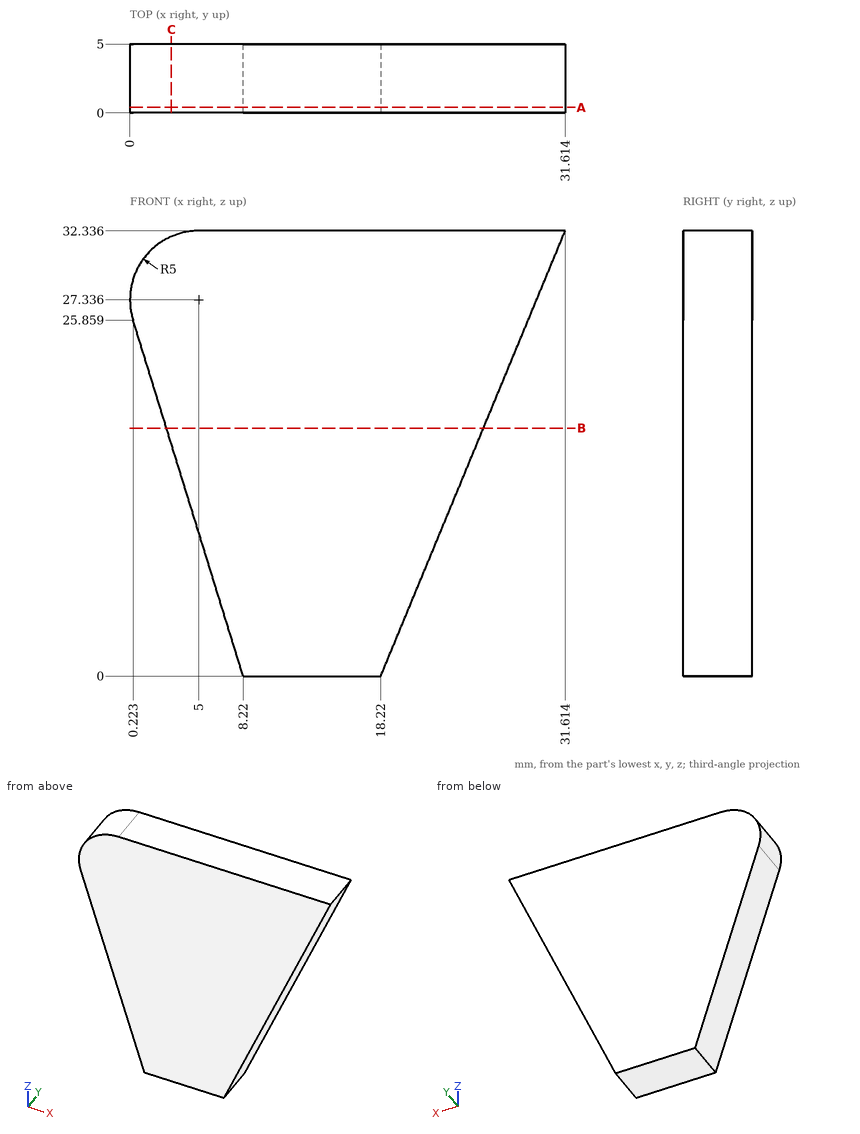
Study the drawing (mm; zero at the part's minimum x, y, z) and answer. Give positions to 0.01 mm unless a question says otherwise; leave off trailing zeros. Write each loop counter-clockwise with the first axis right and the second up, starting at its lowest first coordinate (ties: lowest second). Pieces come first, ordered by that corner, then holes.
(1) Flat-ended cylindrical pins translate along their axes: pin 1 Ø1.5 at (y, z) = (2, 25) entering from -X; pin 2 Ø2 at (y, z) = (4.5, 7.5) entering from +X; pin 3 Ø1 at (y, z) = (3, 8) entering from -X. Find the tip coordinate at first contact, or state that the pin passes through.
Final values:
pin 1: stops at x = 0.26
pin 2: stops at x = 21.74
pin 3: stops at x = 5.59
(2) Straight lines are drawn through the part: line 1 (X direction, y = 1.4, z = 18) (1 decimal); line 2 (Z direction, x = 24.5, y = 2.85) (1 decimal); line 3 (Z direction, x = 22, y = 0.75) (1 decimal). For each, find the intervals that lie inside material, in ascending order.
Final values:
line 1: x = 2.7 to 25.7
line 2: z = 15.2 to 32.3
line 3: z = 9.1 to 32.3
(3) The part is cut by section A-A on y = 0.4. Write down the section's boundary in (x, z) (1 decimal), plus the area to 3 significant figures.
Final values:
outline: (0.2, 25.9) - (8.2, 0) - (18.2, 0) - (31.6, 32.3) - (5, 32.3) arc R5 ccw to start
area: 691 mm2
(4) The part is cut by section B-B on z = 18. Write down the section's boundary in (x, y) (1 decimal).
Final values:
outline: (2.7, 0) - (25.7, 0) - (25.7, 5) - (2.7, 5) - close
(5) The part is cut by section C-C on x = 3. Write down the section's boundary in (y, z), plus the area to 3 significant figures.
Final values:
outline: (0, 16.88) - (5, 16.88) - (5, 31.92) - (0, 31.92) - close
area: 75.2 mm2
